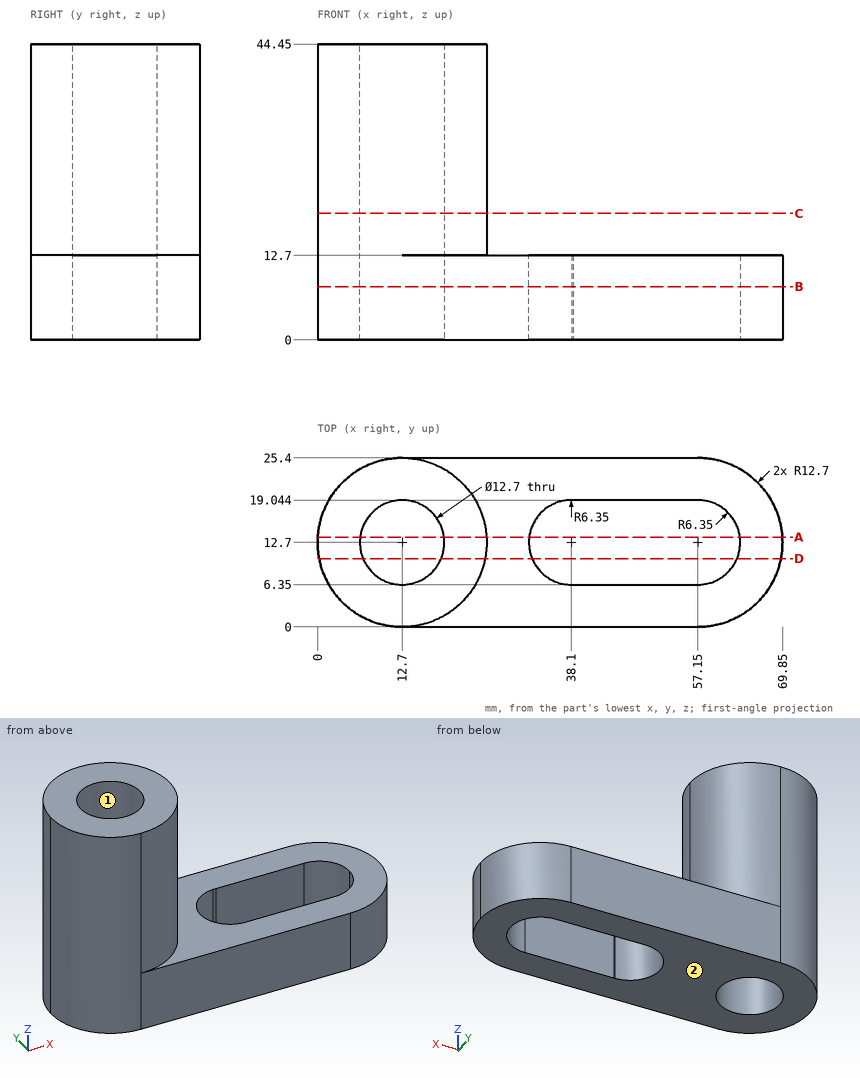
Study the drawing (mm; zero at the part's minimum x, y, z) and answer. Give positions to 0.01 mm unless a question says otherwise; leave off trailing zeros. Order: outer loops, then holes, each group sorted by start corner. A loop starts at its lowest first (then second) coordinate and runs counter-clockwise, first axis right, second up.
1) Find section C-C on z = 19. Write down the section's boundary in (x, y).
Reported:
outline: circle Ø25.4 at (12.7, 12.7); hole circle Ø12.7 at (12.7, 12.7)
2) Given P1, Ø2, axis at y = 5, z = 39, coming from the +X side; P2, Ø12, axis at y = 6, z = 36.5, coming from the -X side; P3, Ø1.5, axis at y = 22.5, z = 32, coming from the -X side, each flat-ended and moving along its own axis, determine where each tip first touches the part or whether it passes through.
Reported:
P1: stops at x = 23.49
P2: stops at x = 0.02
P3: stops at x = 3.79
3) Determine the mould class of the marked faces 1 and 2 for opening direction X: pulls with the +X half, pulls with the -X half, needs draft (parallel to the pull), parting line crosses it, or undercut.
Reported:
face 1: undercut
face 2: needs draft
4) Find section D-D on y = 10.25. Write down the section's boundary in (x, z).
Reported:
outline: (0.24, 0) - (6.84, 0) - (6.84, 44.45) - (0.24, 44.45) - close; (18.56, 0) - (32.24, 0) - (32.24, 12.7) - (25.16, 12.7) - (25.16, 44.45) - (18.56, 44.45) - close; (63.01, 0) - (69.61, 0) - (69.61, 12.7) - (63.01, 12.7) - close
5) Consider line 1 along Y through (x, z) = (12.7, 31.5); line 2 along X through (y, z) = (8.25, 6.5) (1 decimal); line 3 along X through (y, z) = (16.25, 12) (1 decimal). Determine where each line is inside the solid, lowest interval first.
Reported:
line 1: y = 0 to 6.35, 19.05 to 25.4
line 2: x = 0.8 to 8.2, 17.2 to 33.6, 61.7 to 69
line 3: x = 0.5 to 7.4, 18 to 32.8, 62.4 to 69.3
6) Find section B-B on z = 8. Write down the section's boundary in (x, y).
Reported:
outline: (12.7, 0) - (57.15, 0) arc R12.7 ccw to (57.15, 25.4) - (12.7, 25.4) arc R12.7 ccw to start; hole circle Ø12.7 at (12.7, 12.7); hole (38.22, 6.35) - (57.15, 6.35) arc R6.35 ccw to (57.15, 19.05) - (38.38, 19.04) arc R6.35 ccw (long way) to start
7) Find section A-A on y = 13.5. Give the number of separate pieces and of enclosed holes in the cut face, then the cut area to 3 significant figures.
Reported:
separate pieces: 3
enclosed holes: 0
area: 729 mm2
